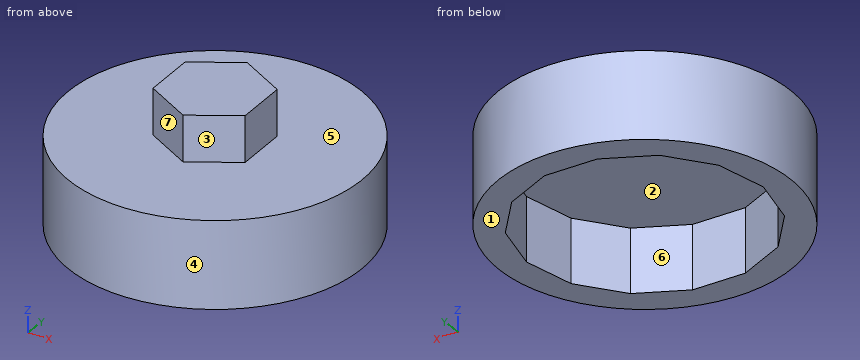
from build123d import *

# Parameters (mm, degrees)
F0_R     = 40.64
F1_DEPTH = 17.78
F2_R     = 40.64
F3_DEPTH = 6.35
F5_DEPTH = 12.7


with BuildPart() as f1:
    # F0 (on Top) → F1 (new body)
    with BuildSketch(Plane.XY):
        Circle(F0_R)
        Polygon((7.391665, -32.385), (-7.391665, -32.385), (-20.710985, -25.970754), (-29.92824, -14.412681), (-33.217841, 0), (-29.92824, 14.412681), (-20.710985, 25.970754), (-7.391665, 32.385), (7.391665, 32.385), (20.710985, 25.970754), (29.92824, 14.412681), (33.217841, 0), (29.92824, -14.412681), (20.710985, -25.970754), align=None, mode=Mode.SUBTRACT)
    extrude(amount=F1_DEPTH)

    # F2 (on face) → F3 (join)
    with BuildSketch(Plane.XY.offset(17.78)):
        Circle(F2_R)
    extrude(amount=F3_DEPTH)

    # F4 (on face) → F5 (join)
    with BuildSketch(Plane.XY.offset(24.13)):
        Polygon((12.497005, 7.673213), (-0.396695, 14.65933), (-12.8937, 6.986117), (-12.497005, -7.673213), (0.396695, -14.65933), (12.8937, -6.986117), align=None)
    extrude(amount=F5_DEPTH)


solid = f1.part
Geometry: final body of the model. Coordinates: model frame, mm. Face numbers are marked on the shaded views. A direction names the side the tool comes from. Round coordinates to 2 decimals unless told otherwise and drop trailing zeros. Order: outer loops, then holes, each group sorted by start corner. A loop starts at its lowest first (then second) coordinate and runs counter-clockwise, first axis right, second up.
Q1. Section A-A, the plane z = 5. Output: boundary loops of the cut face in (x, y) (3 decimals), and give its area (3 significant figures).
Result sheet:
outline: circle Ø81.28 at (0, 0); hole (-33.218, 0) - (-29.928, -14.413) - (-20.711, -25.971) - (-7.392, -32.385) - (7.392, -32.385) - (20.711, -25.971) - (29.928, -14.413) - (33.218, 0) - (29.928, 14.413) - (20.711, 25.971) - (7.392, 32.385) - (-7.392, 32.385) - (-20.711, 25.971) - (-29.928, 14.413) - close
area: 1,840 mm2
Q2. Mould query, pull axis X, two halves, no side actions, for the marked faces 4, 5, 6 and 7. Classes: released by +X, released by -X, zero draft, split by the parting line, or undercut.
Result sheet:
face 4: split by the parting line
face 5: zero draft
face 6: undercut
face 7: released by -X
Q3. Access query for the marked faces 1, 2 and 3. Directions: +Z, -Z, +X, -X, +Y, -Y. A direction counts if a zero-diameter tool reaches every point of the face in a straight line with its end or side. Return the directions, or none.
Result sheet:
face 1: -Z, +X, -X, +Y, -Y
face 2: -Z
face 3: +Z, +X, -Y
Q4. Material intervals for probe 1 along Z at (x, y) = (-32, 4); probe 2 along Y at (x, z) = (26, 15); probe 3 along Y at (x, z) = (-13, 16), sorted ascending.
Result sheet:
probe 1: z = 17.78 to 24.13
probe 2: y = -31.23 to -19.34, 19.34 to 31.23
probe 3: y = -38.5 to -29.68, 29.68 to 38.5
Q5. Pin query (flat end, axial travel): pin 1 (1 mm diameter, centred on y = -31, z = 18.5, fed in from +X); pin 2 (19.5 mm diameter, centred on x = -5, y = -14.5, fed in from -Z); pin 3 (8 mm diameter, centred on x = -17, z = 21, fed in from -Y); pin 4 (24.5 mm diameter, centred on x = -3.5, y = -14.5, fed in from +Z). Return the tip coordinate at first contact, or that it passes through.
Result sheet:
pin 1: stops at x = 26.86
pin 2: stops at z = 17.78
pin 3: stops at y = -38.5
pin 4: stops at z = 36.83
Q6. Section D-D, the plane z = 34.5. Output: boundary loops of the cut face in (x, y), and give its area (3 significant figures).
Result sheet:
outline: (-12.89, 6.99) - (-12.5, -7.67) - (0.4, -14.66) - (12.89, -6.99) - (12.5, 7.67) - (-0.4, 14.66) - close
area: 559 mm2
Q7. Section B-B, the plane x = -32. Output: boundary loops of the cut face in (y, z), and give its area (3 significant figures).
Result sheet:
outline: (-25.05, 0) - (-5.34, 0) - (-5.34, 17.78) - (5.34, 17.78) - (5.34, 0) - (25.05, 0) - (25.05, 24.13) - (-25.05, 24.13) - close
area: 1,020 mm2
Q8. Section C-C, the plane y = -21.5. Output: boundary loops of the cut face in (x, z), and give its area (3 significant figures).
Result sheet:
outline: (-34.49, 0) - (-24.28, 0) - (-24.28, 17.78) - (24.28, 17.78) - (24.28, 0) - (34.49, 0) - (34.49, 24.13) - (-34.49, 24.13) - close
area: 801 mm2
